Autodesk Inventor part; units mm, degrees
ref_plane "YZ Plane" through (0, 0, 0) normal (1, 0, 0) x (0, 1, 0)
ref_plane "XZ Plane" through (0, 0, 0) normal (0, 1, 0) x (-1, 0, 0)
ref_plane "XY Plane" through (0, 0, 0) normal (0, 0, 1) x (1, 0, 0)
sketch "Sketch1" plane through (0, 0, 0) normal (0, 0, 1) x (1, 0, 0)
  line L0 (-79, 15) -> (-76, 15)
  line L1 (-76, 30) -> (-79, 30)
  line L2 (-79, 45) -> (-76, 45)
  line L3 (-76, 60) -> (-79, 60)
  line L4 (-79, 75) -> (-76, 75)
  line L5 (-76, 90) -> (-79, 90)
  line L6 (76, 15) -> (79, 15)
  line L7 (76, 30) -> (79, 30)
  line L8 (79, 45) -> (76, 45)
  line L9 (76, 60) -> (79, 60)
  line L10 (79, 75) -> (76, 75)
  line L11 (79, 90) -> (76, 90)
  line L12 (-56.4286, 0) -> (-56.4286, 3)
  line L13 (-33.8571, 3) -> (-33.8571, 0)
  line L14 (-11.2857, 0) -> (-11.2857, 3)
  line L15 (11.2857, 0) -> (11.2857, 3)
  line L16 (33.8571, 0) -> (33.8571, 3)
  line L17 (56.4286, 0) -> (56.4286, 3)
  line L18 (-56.4286, 102) -> (-56.4286, 105)
  line L19 (-33.8571, 102) -> (-33.8571, 105)
  line L20 (-11.2857, 102) -> (-11.2857, 105)
  line L21 (11.2857, 102) -> (11.2857, 105)
  line L22 (33.8571, 102) -> (33.8571, 105)
  line L23 (56.4286, 102) -> (56.4286, 105)
  line L24 (-56.4286, 3) -> (-76, 3)
  line L25 (-76, 3) -> (-76, 15)
  line L26 (-76, 30) -> (-76, 45)
  line L27 (-76, 60) -> (-76, 75)
  line L28 (-76, 90) -> (-76, 102)
  line L29 (-76, 102) -> (-56.4286, 102)
  line L30 (-33.8571, 102) -> (-11.2857, 102)
  line L31 (11.2857, 102) -> (33.8571, 102)
  line L32 (56.4286, 102) -> (76, 102)
  line L33 (-11.2857, 3) -> (-33.8571, 3)
  line L34 (76, 3) -> (56.4286, 3)
  line L35 (33.8571, 3) -> (11.2857, 3)
  line L36 (-79, 75) -> (-79, 90)
  line L37 (-79, 15) -> (-79, 30)
  line L38 (-79, 45) -> (-79, 60)
  line L39 (-33.8571, 0) -> (-56.4286, 0)
  line L40 (56.4286, 0) -> (33.8571, 0)
  line L41 (11.2857, 0) -> (-11.2857, 0)
  line L42 (-56.4286, 105) -> (-33.8571, 105)
  line L43 (-11.2857, 105) -> (11.2857, 105)
  line L44 (33.8571, 105) -> (56.4286, 105)
  line L45 (79, 30) -> (79, 15)
  line L46 (79, 90) -> (79, 75)
  line L47 (79, 60) -> (79, 45)
  line L48 (76, 102) -> (76, 90)
  line L49 (76, 75) -> (76, 60)
  line L50 (76, 45) -> (76, 30)
  line L51 (76, 15) -> (76, 3)
  point P0 (0, 0)
  dimension "d1" = 158
  dimension "d5" = 22.5714
  dimension "d6" = 79
  dimension "d7" = 45.1429
  dimension "d8" = 67.7143
  dimension "d9" = 90.2857
  dimension "d10" = 112.8571
  dimension "d11" = 135.4286
  dimension "d12" = 105
  dimension "d13" = 15
  dimension "d14" = 0
  dimension "d15" = 3
  dimension "d16" = 30
  dimension "d17" = 45
  dimension "d18" = 60
  dimension "d19" = 75
  dimension "d20" = 90
  dimension "d21" = 99
  dimension "d22" = 3
  dimension "d23" = 3
extrude "Extrusion1" add sketch "Sketch1" along normal blind 3
equation "\"d1\" = shelfWs"
equation "\"d5\" = 0.142857 * shelfWs - tol"
equation "\"d7\" = 0.285714 * shelfWs + tol"
equation "\"d8\" = 0.428571 * shelfWs - tol"
equation "\"d9\" = 0.571429 * shelfWs + tol"
equation "\"d10\" = 0.714286 * shelfWs - tol"
equation "\"d11\" = 0.857143 * shelfWs + tol"
equation "\"d13\" = 0.142857 * shelfD - tol"
equation "\"d15\" = tt"
equation "\"d16\" = 0.285714 * shelfD + tol"
equation "\"d17\" = 0.428571 * shelfD - tol"
equation "\"d18\" = 0.571429 * shelfD + tol"
equation "\"d19\" = 0.714286 * shelfD - tol"
equation "\"d20\" = 0.857143 * shelfD + tol"
equation "\"d21\" = -2 * tt + shelfD"
equation "\"d22\" = tt"
equation "\"d23\" = tt"
equation "\"d24\" = tt"
equation "\"d0\" = 0.5 * shelfWs"
equation "\"tt\" = 3"
equation "\"tol\" = 0"
equation "\"d2\" = shelfD"
equation "\"d4\" = tt"
equation "\"tiroir\" = 1"
equation "\"nHoles\" = 4"
equation "\"shelfH\" = 35"
properties part number "back"
Geometry check sheet. Reference: the model listing, model coordinates, mm. A direction names the side the tool comes from. Coordinates: 2 decimals unless noted, no trailing zeros. Order: outer loops, then holes, each group sorted by start corner. A loop starts at its lowest first (then second) coordinate and runs counter-clockwise, first axis right, second up. Notation, with made-up numbers: (30, 16) - (65, 16) arc R21 ccw to (65, 39) - close; hole circle Ø7 at (66.5, 80). An arc over 180 degrees is marked (long way). Answer in a Markdown table with one row per item. Add a question column.
1) Gauge pin test, flat ends, axial feed: P1, Ø1.5, axis at x = -77, z = 2, coming from the -Y side; P2, Ø1.5, axis at x = -69.5, z = 1.5, coming from the -Y side; P3, Ø1.5, axis at y = 103, z = 1, coming from the +X side. Record the tip position at first contact, or that the pin passes through.
2) Material ranges on line 1 along Y through (x, z) = (-69.5, 1.65); line 2 along X through (y, z) = (73, 2.25), recorded low to high. Write a range as [from, to].
3) Set-up check for faces 1 (the flat face through (-77, 90, 1)), 2 (the flat face through (76, 96, 1)), 3 (the flat face through (-76, 67, 1)), 4 (the flat face through (11.286, 103, 1)): record each of +Z, -Z, +X, -X, +Y, -Y from which the full face is reachable in a straight line by a thin tool's end or side.
4) Cross-section at A-A, the plane y = 98. Record the cut outline in (x, z), then the cut area to 3 significant figures.
5) Cross-section at B-B, the plane x = 64. Record the cut outline in (y, z), then the cut area to 3 significant figures.
6) Release check for a two-part mould opening along Y. For faces 5 (the flat face through (77, 15, 1)), 6 (the flat face through (78, 45, 1)), 7 (the flat face through (-56.429, 103, 1)) record: +Y half, -Y half, draft (parallel to the pull), parting line (faces both ways), or undercut.
Check result:
| question | item | result |
|---|---|---|
| 1 | P1 | stops at y = 15 |
| 1 | P2 | stops at y = 3 |
| 1 | P3 | stops at x = 56.43 |
| 2 | line 1 | y = [3, 102] |
| 2 | line 2 | x = [-76, 76] |
| 3 | face 1 | +Z, -Z, -X, +Y |
| 3 | face 2 | +Z, -Z, +X, +Y |
| 3 | face 3 | +Z, -Z, -X |
| 3 | face 4 | +Z, -Z, +Y |
| 4 | outline | (-76, 0) - (76, 0) - (76, 3) - (-76, 3) - close |
| 4 | area | 456 mm² |
| 5 | outline | (3, 0) - (102, 0) - (102, 3) - (3, 3) - close |
| 5 | area | 297 mm² |
| 6 | face 5 | -Y half |
| 6 | face 6 | undercut |
| 6 | face 7 | draft |
